```python
from build123d import *

# Parameters (mm, degrees)
SKETCH_6_W               = 4
SKETCH_6_H               = 9.6
CUT_EXTRUDE_4_DEPTH      = 84.366660003
SKETCH_7_R               = 12
CUT_EXTRUDE_7_DEPTH      = 80.837334625
PATTERN_CIRCULAR_2_COUNT = 6


with BuildPart() as part:
    # Sketch 5 → Revolve 4 (revolve)
    with BuildSketch(Plane.XY, mode=Mode.PRIVATE) as revolve_4_sk:
        Polygon((-15.948135722, 7.5), (14.051864278, 7.5), (14.051864278, 16), (2.051864278, 16), (2.051864278, 45), (10.051864278, 45), (10.051864278, 55), (6.995140411, 55), (5.273502344, 50), (2.273502344, 50), (0.551864278, 55), (-2.448135722, 55), (-4.169773789, 50), (-7.169773789, 50), (-8.891411855, 55), (-11.948135722, 55), (-11.948135722, 45), (-3.948135722, 45), (-3.948135722, 16), (-15.948135722, 16), align=None)
    revolve(revolve_4_sk.sketch.rotate(Axis((-49.922793891, 0, 0), (1, 0, 0)), 90), axis=Axis((-49.922793891, 0, 0), (1, 0, 0)))

    # Sketch 6 → Cut-Extrude 4 (cut, through all)
    with BuildSketch(Plane(origin=(14.051864278, 0, 0), x_dir=(0, 0, -1), z_dir=(1, 0, 0))):
        with Locations((0, 4.8)):
            Rectangle(SKETCH_6_W, SKETCH_6_H)
    extrude(amount=-CUT_EXTRUDE_4_DEPTH, mode=Mode.SUBTRACT)

    # Sketch 7 → Cut-Extrude 7 (cut, through all)
    with BuildSketch(Plane.ZY.offset(3.948135722)):
        with Locations((0, 30)):
            Circle(SKETCH_7_R)
    cut_extrude_7 = extrude(amount=-CUT_EXTRUDE_7_DEPTH, mode=Mode.SUBTRACT)

    # Pattern Circular 2: Cut-Extrude 7 ×6 about axis
    pattern_circular_2_axis = Axis((0, 0, 0), (1, 0, 0))
    for i in range(1, PATTERN_CIRCULAR_2_COUNT):
        add(cut_extrude_7.rotate(pattern_circular_2_axis, i * 360 / PATTERN_CIRCULAR_2_COUNT), mode=Mode.SUBTRACT)


solid = part.part
```
Geometry check sheet. Reference: the model listing, model coordinates, mm. A direction names the side the tool comes from. Coordinates: 2 decimals unless noted, no trailing zeros. Order: outer loops, then holes, each group sorted by start corner. A loop starts at its lowest first (then second) coordinate and runs counter-clockwise, first axis right, second up. Notation, with made-up numbers: (-2.75, 53.25) - (16.25, 53.25) arc R28 ccw to (16.25, 88.25) - close; hole circle Ø5 at (75, 53.25). An arc over 180 degrees is marked (long way). Answer as a JSON object with one key per item and string values. Group by question number.
Item 1: Sectioned sample at A-A, the plane x = 8.5. Record the cut outline in (y, z), and give its area (3 significant figures).
Item 2: Scan lines: probe 1 along Y at (x, z) = (0, 0); probe 2 along Y at (x, z) = (2.5, -4); probe 3 along Y at (x, z) = (5, 12.5). Record each from-to range of solid material in increasing order.
Item 3: Depth check by flat-ended pin: pin 1 Ø4 at (y, z) = (25.5, -19.5) entering from +X; pin 2 Ø1 at (x, z) = (8.5, 18.5) entering from +Y; pin 3 Ø6 at (x, y) = (7.5, 30.5) entering from +Z. Enter the tip coordinate at first touch or a pass-through.
Item 4: Tool access check on faces 1 (the face through (2.052, -1, -19)), 2 (the face through (-3.948, -1, 19)), 3 (the face through (3.75, -15.02, 47.69)). Record the directions out of +Z, -Z, +X, -X, +Y, -Y that give a thin tool (end or side, any length) a straight path to the whole face; none if there is none.
Item 5: Sectioned sample at B-B, the plane z = 0. Give the number of separate pieces and of enclosed holes in the cut face, and give its area (3 significant figures).
Item 6: Draft check along Y on faces 4 (the face through (-7.28, 49.12, -10.91)), 5 (the face through (-0.99, 14.472, -13.992)), 6 (the face through (-15.948, 3.33, 6.89)). Enter one of: +Y half, -Y half, draft (parallel to the pull), parting line (faces both ways), or undercut.
Resolved:
{
 "1": {"outline": "circle Ø110 at (0, 0); circle Ø32 at (0, 0); hole circle Ø90 at (0, 0); hole (7.23, -2) - (9.6, -2) - (9.6, 2) - (7.23, 2) arc R7.5 ccw (long way) to start", "area": "3,760 mm^2"},
 "2": {"probe 1": "-55 to -42, -18 to -7.5, 9.6 to 18, 42 to 55", "probe 2": "-49.84 to -44.82, -15.49 to -6.34, 6.34 to 15.49, 44.82 to 49.84", "probe 3": "-48.41 to -43.23, -9.99 to 9.99, 43.23 to 48.41"},
 "3": {"pin 1": "x = 2.05", "pin 2": "y = 51.97", "pin 3": "z = 47.63"},
 "4": {"face 1": "+X", "face 2": "-X", "face 3": "none"},
 "5": {"separate pieces": "4", "enclosed holes": "0", "area": "853 mm^2"},
 "6": {"face 4": "parting line", "face 5": "undercut", "face 6": "draft"}
}
